```python
from build123d import *

# Parameters (mm, degrees)
SKETCH_W            = 34.6
SKETCH_H            = 24.6
PAD001_DEPTH        = 1
SKETCH002_R         = 1.016
PAD002_DEPTH        = 5
LINEARPATTERN_COUNT = 2
LINEARPATTERN_PITCH = 17.9


with BuildPart() as part:
    # Sketch → Pad001 (new body)
    with BuildSketch(Plane.XY):
        Rectangle(SKETCH_W, SKETCH_H)
    extrude(amount=PAD001_DEPTH)

    # Sketch002 → Pad002 (join)
    with BuildSketch(Plane.XY):
        with Locations((-2.484719, -9.134)):
            Circle(SKETCH002_R)
        Polygon((-11.875322, 9.261), (-10.815853, 10.15), (-3.50471, 10.15), (-2.75875, 9.261), (-3.818219, 8.372), (-11.129362, 8.372), align=None)
        Polygon((-12.171581, 9.021337), (-11.425621, 8.132337), (-12.643997, 1.222585), (-13.703466, 0.333585), (-14.449425, 1.222585), (-13.23105, 8.132337), align=None)
        Polygon((-2.56357, 8.927415), (-3.623039, 8.038415), (-4.841415, 1.128663), (-4.095455, 0.239663), (-3.035986, 1.128663), (-1.81761, 8.038415), align=None)
        Polygon((-12.448817, 0.889), (-13.508286, 0), (-12.762326, -0.889), (-5.451183, -0.889), (-4.391714, 0), (-5.137674, 0.889), align=None)
        Polygon((-13.804545, -0.239663), (-14.864014, -1.128663), (-16.08239, -8.038415), (-15.33643, -8.927415), (-14.276961, -8.038415), (-13.058585, -1.128663), align=None)
        Polygon((-4.196534, -0.333585), (-5.256003, -1.222585), (-6.474379, -8.132337), (-5.728419, -9.021337), (-4.66895, -8.132337), (-3.450575, -1.222585), align=None)
        Polygon((-15.14125, -9.261), (-14.081781, -8.372), (-6.770638, -8.372), (-6.024678, -9.261), (-7.084147, -10.15), (-14.39529, -10.15), align=None)
    pad002 = extrude(amount=PAD002_DEPTH)

    # LinearPattern: Pad002 ×2
    with Locations(*[(i * LINEARPATTERN_PITCH, 0, 0) for i in range(1, LINEARPATTERN_COUNT)]):
        add(pad002)


with BuildPart() as part_1:
    # Body001 placement: moved
    add(part.part.moved(Location((0, 0, 5))))


solid = part_1.part
```
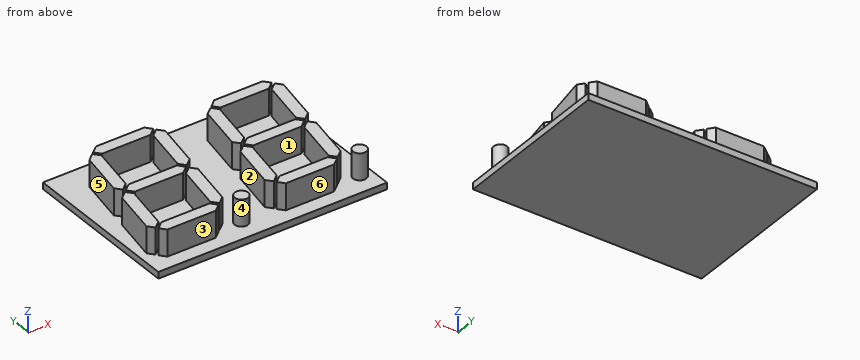
Source: CAD feature listing. Evaluate the final solid. Frame: model axes, mm. Face numbers are marked on the shaded views. A direction names the side the tool comes from. Give positions to 0.01 mm unless a question says otherwise; leave off trailing zeros. Order: outer loops, then holes, each group sorted by start corner. A loop starts at its lowest first (then second) coordinate and runs counter-clockwise, first axis right, second up. Notation, with made-up numbers: (16, -23.75) -> (58, -23.75) arc R21 ccw to (58, -1.75) -> close; hole circle Ø3 at (60.5, 59). An arc over 180 degrees is marked (long way). Use a Markdown table: item, result.
Q1. Section A-A (x = -8.5). Return the cut outline in (y, z), and give its area (3 significant figures).
A:
| item | result |
|---|---|
| outline | (-12.3, 5) -> (12.3, 5) -> (12.3, 6) -> (10.15, 6) -> (10.15, 10) -> (8.37, 10) -> (8.37, 6) -> (0.89, 6) -> (0.89, 10) -> (-0.89, 10) -> (-0.89, 6) -> (-8.37, 6) -> (-8.37, 10) -> (-10.15, 10) -> (-10.15, 6) -> (-12.3, 6) -> close |
| area | 45.9 mm^2 |
Q2. Section D-D (x = -0.5). Return the cut outline in (y, z), and give its area (3 significant figures).
A:
| item | result |
|---|---|
| outline | (-12.3, 5) -> (12.3, 5) -> (12.3, 6) -> (-12.3, 6) -> close |
| area | 24.6 mm^2 |
Q3. Section B-B (y = 6.25). Return the cut outline in (x, z).
A:
| item | result |
|---|---|
| outline | (-17.3, 5) -> (17.3, 5) -> (17.3, 6) -> (15.77, 6) -> (15.77, 10) -> (13.96, 10) -> (13.96, 6) -> (6.14, 6) -> (6.14, 10) -> (4.34, 10) -> (4.34, 6) -> (-2.13, 6) -> (-2.13, 10) -> (-3.94, 10) -> (-3.94, 6) -> (-11.76, 6) -> (-11.76, 10) -> (-13.56, 10) -> (-13.56, 6) -> (-17.3, 6) -> close |
Q4. First-contact query: P1, Ø4, axis at x = 6.5, y = 5.5, coming from the +Z side; P2, Ø1.5, axis at y = 2, z = 7, coming from the +X side; P3, Ø1.2, axis at x = -11.5, z = 7, coming from the -Y side; P4, Ø1.2, axis at x = -9, z = 7, coming from the +Y side. Flat tips, straight axial feed; report the tip coordinate or a pass-through.
A:
| item | result |
|---|---|
| P1 | z = 10 |
| P2 | x = 15.15 |
| P3 | y = -10.15 |
| P4 | y = 10.15 |
Q5. Material intervals for line 1 (Y direction, x = -10.5, z = 7.55); line 2 (X direction, y = 5.25, z = 8.65); line 3 (X direction, y = 7.5, z = 8.2), sorted ascending. Write a range as [from, to].
A:
| item | result |
|---|---|
| line 1 | [-10.15, -8.37], [-0.89, 0.89], [8.37, 10.15] |
| line 2 | [-13.74, -11.93], [-4.11, -2.31], [4.16, 5.97], [13.79, 15.59] |
| line 3 | [-13.34, -11.54], [-3.72, -1.91], [4.56, 6.36], [14.18, 15.99] |
Q6. Access query for the marked faces 1, 2 and 3. Directions: +Z, -Z, +X, -X, +Y, -Y. A direction counts if a zero-diameter tool reaches every point of the face in a straight line with its end or side. Return the directions, or none.
A:
| item | result |
|---|---|
| face 1 | +Z |
| face 2 | +Z, +Y |
| face 3 | +Z, +X, -X, -Y |
Q7. Section C-C (z = 7.35). State how many separate pieces and enclosed holes the cut face has, and give its area (3 significant figures).
A:
| item | result |
|---|---|
| separate pieces | 16 |
| enclosed holes | 0 |
| area | 207 mm^2 |
Q8. Pull-direction query (Y, two-part tool) for the marked faces 4, 5 and 6; classes: +Y half, -Y half, draft (parallel to the pull), parting line (faces both ways), or undercut.
A:
| item | result |
|---|---|
| face 4 | undercut |
| face 5 | +Y half |
| face 6 | -Y half |
